from build123d import *

# Parameters (mm, degrees)
SKETCH1_R           = 1.5
BOSS_EXTRUDE1_DEPTH = 1.6
BOSS_EXTRUDE2_DEPTH = 2.3


with BuildPart() as part:
    # Sketch1 → Boss-Extrude1 (new body)
    with BuildSketch(Plane.XY):
        Polygon((-65.182649766, 43.872204631), (-65.182649766, 36.172204631), (-72.882649766, 36.172204631), (-72.882649766, -46.427795369), (-65.182649766, -46.427795369), (-65.182649766, -54.127795369), (17.417350234, -54.127795369), (17.417350234, -46.427795369), (25.117350234, -46.427795369), (25.117350234, 36.172204631), (17.417350234, 36.172204631), (17.417350234, 43.872204631), align=None)
        with Locations((-69.882649766, 19.572204631)):
            Circle(SKETCH1_R, mode=Mode.SUBTRACT)
        with Locations((-69.882649766, -29.827795369)):
            Circle(SKETCH1_R, mode=Mode.SUBTRACT)
        with Locations((-48.582649766, -51.127795369)):
            Circle(SKETCH1_R, mode=Mode.SUBTRACT)
        with Locations((0.817350234, -51.127795369)):
            Circle(SKETCH1_R, mode=Mode.SUBTRACT)
        with Locations((22.117350234, -29.827795369)):
            Circle(SKETCH1_R, mode=Mode.SUBTRACT)
        with Locations((22.117350234, 19.572204631)):
            Circle(SKETCH1_R, mode=Mode.SUBTRACT)
        with Locations((0.817350234, 40.872204631)):
            Circle(SKETCH1_R, mode=Mode.SUBTRACT)
        with Locations((-48.582649766, 40.872204631)):
            Circle(SKETCH1_R, mode=Mode.SUBTRACT)
        Polygon((-63.382649766, 22.222204631), (-50.382649766, 35.222204631), (2.617350234, 35.222204631), (15.617350234, 22.222204631), (15.617350234, -5.077795369), (-63.382649766, -5.077795369), align=None, mode=Mode.SUBTRACT)
        Polygon((-63.382649766, -18.177795369), (-50.382649766, -5.177795369), (2.617350234, -5.177795369), (15.617350234, -18.177795369), (15.617350234, -45.477795369), (-63.382649766, -45.477795369), align=None, mode=Mode.SUBTRACT)
    extrude(amount=BOSS_EXTRUDE1_DEPTH)

    # Sketch1_3 → Boss-Extrude2 (add)
    with BuildSketch(Plane.XY):
        Polygon((-63.382649766, -5.077795369), (-63.382649766, 22.222204631), (-50.382649766, 35.222204631), (2.617350234, 35.222204631), (15.617350234, 22.222204631), (15.617350234, -5.077795369), align=None)
        Polygon((-63.382649766, -18.177795369), (-50.382649766, -5.177795369), (2.617350234, -5.177795369), (15.617350234, -18.177795369), (15.617350234, -45.477795369), (-63.382649766, -45.477795369), align=None)
    extrude(amount=BOSS_EXTRUDE2_DEPTH)


solid = part.part
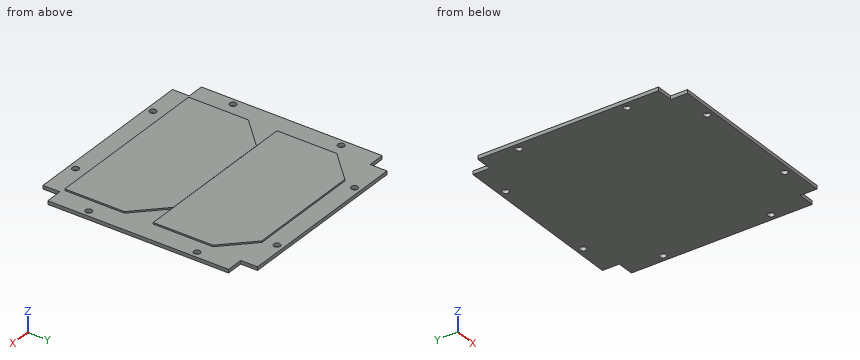
Here's how the part is built. I have some questions about the finished solid (model axes, mm). Round coordinates to 2 decimals unless told otherwise and drop trailing zeros. Order: outer loops, then holes, each group sorted by start corner. A loop starts at its lowest first (then second) coordinate and runs counter-clockwise, first axis right, second up. Notation, with made-up numbers: (60, 30.25) -> (87, 30.25) arc R27 cw to (87, 65.25) -> close; hole circle Ø5 at (33.5, -1.75). An arc over 180 degrees is marked (long way). Return JSON: item names as keys, results as strings.
Q1. For pin 1 Ø0.6 at (y, z) = (8, 2) entering from +X; pin 2 Ø5 at (x, y) = (22.12, -29.83) entering from +Z; pin 3 Ø0.6 at (x, z) = (-30.5, 2) entering from -Y, each with a flat end and sliding along its axis, tell me the tip position at first contact or that it passes through.
Filled sheet:
{"pin 1": "stops at x = 15.62", "pin 2": "stops at z = 1.6", "pin 3": "stops at y = -45.48"}
Q2. If we section it at B-B on z = 0.85: Give the number of separate pieces and of enclosed holes in the cut face, plus the area to 3 significant figures.
Filled sheet:
{"separate pieces": "1", "enclosed holes": "8", "area": "9,310 mm^2"}
Q3. If we section it at D-D on y = 31: List the corners of the cut face in (x, z) for me.
Filled sheet:
{"outline": "(-72.88, 0) -> (25.12, 0) -> (25.12, 1.6) -> (6.84, 1.6) -> (6.84, 2.3) -> (-54.6, 2.3) -> (-54.6, 1.6) -> (-72.88, 1.6) -> close"}
Q4. If we section it at C-C on x = -21: List the corners of the cut face in (y, z) for me.
Filled sheet:
{"outline": "(-54.13, 0) -> (43.87, 0) -> (43.87, 1.6) -> (35.22, 1.6) -> (35.22, 2.3) -> (-5.08, 2.3) -> (-5.08, 1.6) -> (-5.18, 1.6) -> (-5.18, 2.3) -> (-45.48, 2.3) -> (-45.48, 1.6) -> (-54.13, 1.6) -> close"}
Q5. I need wall thicknesses on line 1 along Y through (x, z) = (-68, 1.2); line 2 along Y through (x, z) = (-55.5, 1.8); line 3 along Z through (x, y) = (-63, -14.5). Which ranges of each line are inside material? Lowest first, please. Write a range as from..to.
Filled sheet:
{"line 1": "y = -46.43..36.17", "line 2": "y = -45.48..-10.3, -5.08..30.1", "line 3": "z = 0..1.6"}
Q6. If we section it at A-A on y = -3.5: List the corners of the cut face in (x, z) for me, plus the area to 3 significant figures.
Filled sheet:
{"outline": "(-72.88, 0) -> (25.12, 0) -> (25.12, 1.6) -> (15.62, 1.6) -> (15.62, 2.3) -> (-63.38, 2.3) -> (-63.38, 1.6) -> (-72.88, 1.6) -> close", "area": "212 mm^2"}
